Study the drawing (mm; zero at the part's minimum x, y, z) and answer. A direction names the side the tool comes from. Coordinates: 2 decimals unless noted, no trailing zeros. Loops run counter-clockwise (first coordinate to the right, second up) from the corner with the lowest first, then second, coordinate; pieces in that order, holes last. Notation, with made-up numbers: M 74,58 L 117,58 A17 cw 117,64 Z; hole C 28,-16 d7. An arc over 180 degrees is marked long. Use one line per item in the form item = value. Start each with the question number.
1. The part is cut by section D-D (y = 4.5). Give the vertices of the cut face in (x, z).
2. A tool of negligible diameter and unlimited length cuts with its end or side. For the marked faces 1, 2 and 3, from which of +Z, -Z, +X, -X, +Y, -Y can it reach the whole face along a straight path? Write none if from no direction.
3. Flat-ended cylindrical pins translate along their axes: pin 1 (1.3 mm diameter, centred on y = 10, z = 9.5, fed in from +X); pin 2 (1.2 mm diameter, centred on y = 5.5, z = 26, fed in from +X); pin 3 (6 mm diameter, centred on y = 2.5, z = 6, fed in from -X); pin 4 (0.8 mm diameter, centred on x = 15, z = 26, fed in from -Y). Find the tip coordinate at first contact, or state that the pin passes through.
4. The part is cut by section B-B (x = 14.75). Give the vertices of the cut face in (y, z).
5. The part is cut by section C-C (z = 7). Give the vertices of the cut face in (x, y).
6. The part is cut by section A-A (z = 2.05). Give the vertices of the cut face in (x, y).
7. Find the intervals of material crossed by probe 1 along Z at (x, y) = (2.25, 8.5) (1 decimal); probe 2 along Y at (x, z) = (5.5, 16.5); probe 3 along Z at (x, y) = (13.5, 3.5), in increasing order. Write a range as [from, to].
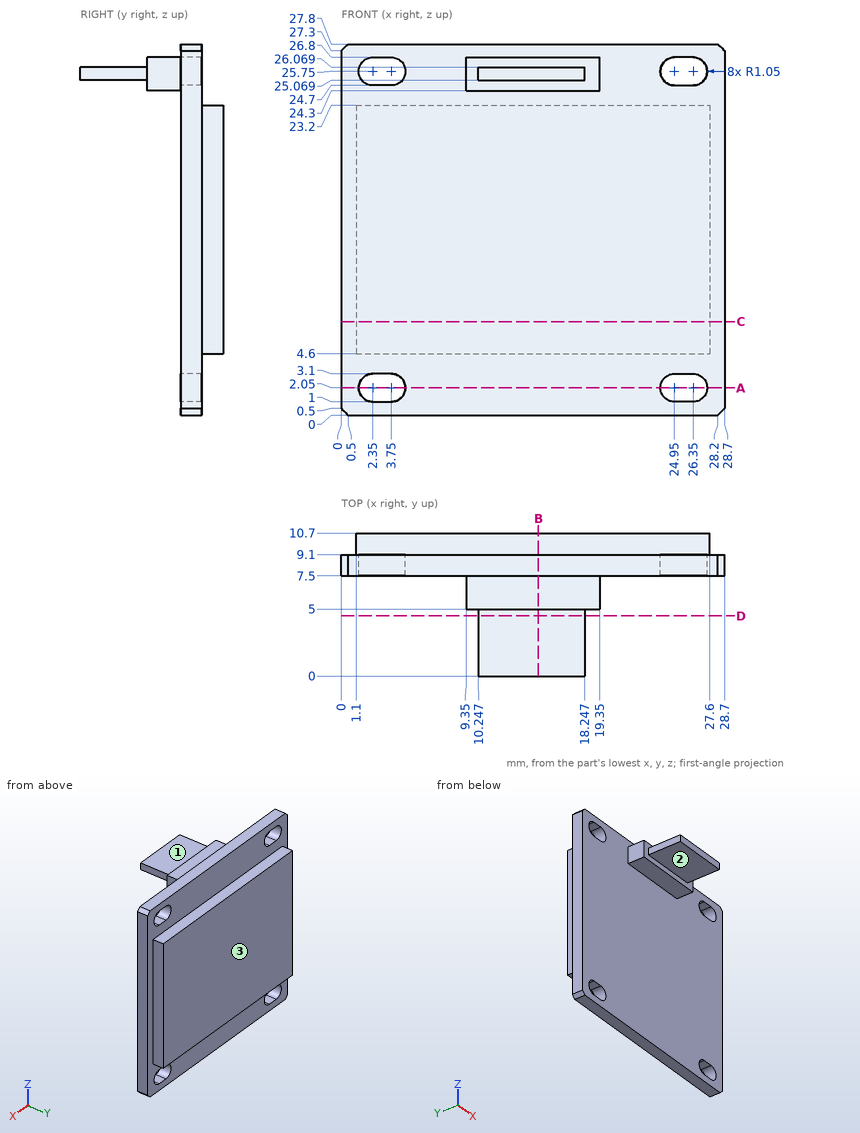
Computed values:
q1.outline = M 10.25,25.07 L 18.25,25.07 L 18.25,26.07 L 10.25,26.07 Z
q2.face_1 = +Z, +X, -X, -Y
q2.face_2 = -Z, +X, -X, -Y
q2.face_3 = +Z, -Z, +X, -X, +Y
q3.pin_1 = 27.6
q3.pin_2 = 19.35
q3.pin_3 = through
q3.pin_4 = 0
q4.outline = M 0,25.07 L 5,25.07 L 5,24.3 L 7.5,24.3 L 7.5,0 L 9.1,0 L 9.1,4.6 L 10.7,4.6 L 10.7,23.2 L 9.1,23.2 L 9.1,27.8 L 7.5,27.8 L 7.5,26.8 L 5,26.8 L 5,26.07 L 0,26.07 Z
q5.outline = M 0,7.5 L 28.7,7.5 L 28.7,9.1 L 27.6,9.1 L 27.6,10.7 L 1.1,10.7 L 1.1,9.1 L 0,9.1 Z
q6.outline = M 0,7.5 L 1.3,7.5 L 1.3,9.1 L 0,9.1 Z; M 4.8,7.5 L 23.9,7.5 L 23.9,9.1 L 4.8,9.1 Z; M 27.4,7.5 L 28.7,7.5 L 28.7,9.1 L 27.4,9.1 Z
q7.probe_1 = [0, 1], [3.1, 24.7], [26.8, 27.8]
q7.probe_2 = [7.5, 10.7]
q7.probe_3 = [25.07, 26.07]
